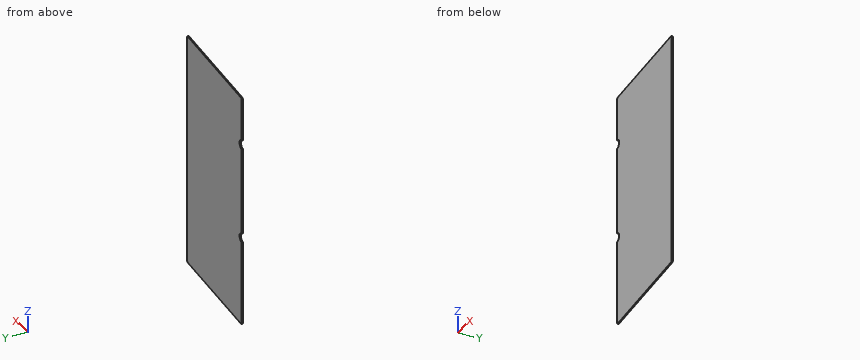
```python
from build123d import *

# Parameters (mm, degrees)
BOSS_EXTRUDE1_DEPTH = 1168.4
SKETCH4_R           = 22.225
CUT_EXTRUDE1_DEPTH  = 58.348513463
FILLET1_R           = 6.35


with BuildPart() as part:
    # Sketch1 → Boss-Extrude1 (new body)
    with BuildSketch(Plane.XY):
        Polygon((22.225, 51.193319499), (607.367319431, 0), (607.920758397, 6.325836333), (22.778438966, 57.519155832), align=None)
    extrude(amount=BOSS_EXTRUDE1_DEPTH)

    # Sketch4 → Cut-Extrude1 (cut, through all)
    with BuildSketch(Plane(origin=(5.167076131, 59.05995043, 0), x_dir=(0.996194698, -0.087155743, 0), z_dir=(0.087155743, 0.996194698, 0))):
        with Locations((17.67863538, -446.88125)):
            Circle(SKETCH4_R)
        with Locations((17.67863538, -927.89375)):
            Circle(SKETCH4_R)
    extrude(amount=-CUT_EXTRUDE1_DEPTH, mode=Mode.SUBTRACT)

    # Fillet1
    fillet1_edges = [part.edges().sort_by_distance(p)[0] for p in [
        (607.644038914, 3.162918166, 1168.4),
        (22.501719483, 54.356237666, 1168.4),
        (607.644038914, 3.162918166, 0),
        (22.501719483, 54.356237666, 0),
    ]]
    fillet(fillet1_edges, radius=FILLET1_R)


solid = part.part
```
Work out the finished part from the listing and answer in its coordinate system (mm). Coordinates: 2 decimals unless noted, no trailing zeros. Write each loop counter-clockwise with the first axis right and the second up, starting at its lowest first coordinate (ties: lowest second). Pieces come first, ordered by that corner, then holes. Notation, with made-up numbers: (39, 70.25) - (86, 70.25) arc R6 cw to (86, 79.25) - close; hole circle Ø7 at (-16, 13). An arc over 180 degrees is marked (long way). Answer as a JSON object with one key per item and string values.
Q1. Consider L1, parallel to Y at x = 509.5, z = 385; L2, parallel to Y at x = 280, z = 908. Determine where each line is inside the solid, lowest interval first. Write a range as from..to.
Results list:
{"L1": "y = 8.56..14.94", "L2": "y = 28.64..35.02"}
Q2. Find section A-A (z = 366). Write down the section's boundary in (x, y) (3 decimals), plus the area to 3 significant figures.
Results list:
{"outline": "(22.225, 51.193) - (607.367, 0) - (607.921, 6.326) - (22.778, 57.519) - close", "area": "3,730 mm^2"}
Q3. Given pin 1 Ø1.5 at (x, z) = (536.5, 627.5) entering from +Y; pin 2 Ø6 at (x, z) = (298, 848) entering from -Y; pin 3 Ø10 at (x, z) = (140, 784) entering from -Y, each flat-ended and moving along its own axis, determine where each tip first touches the part or whether it passes through.
Results list:
{"pin 1": "stops at y = 12.64", "pin 2": "stops at y = 26.8", "pin 3": "stops at y = 40.45"}
Q4. Find section B-B (y = 19). Write down the section's boundary in (x, z), plus the area to 3 significant figures.
Results list:
{"outline": "(390.2, 0) - (463.05, 0) - (463.05, 1168.4) - (390.2, 1168.4) - close", "area": "85,100 mm^2"}
